```python
from build123d import *

# Parameters (mm, degrees)
SKETCH_1_R      = 8
SKETCH_1_R_2    = 1.56
EXTRUDE_1_DEPTH = 3


with BuildPart() as part:
    # 草图1 → 凸台-拉伸1 (new body)
    with BuildSketch(Plane.XY):
        with BuildLine():
            Line((-27.357864376, 42), (27.357864376, 42))
            ThreePointArc((27.357864376, 42), (31.1846987, 41.238795325), (34.428932188, 39.071067812))
            Line((34.428932188, 39.071067812), (39.071067812, 34.428932188))
            ThreePointArc((39.071067812, 34.428932188), (41.238795325, 31.1846987), (42, 27.357864376))
            Line((42, 27.357864376), (42, -27.357864376))
            ThreePointArc((42, -27.357864376), (41.238795325, -31.1846987), (39.071067812, -34.428932188))
            Line((39.071067812, -34.428932188), (34.428932188, -39.071067812))
            ThreePointArc((34.428932188, -39.071067812), (31.1846987, -41.238795325), (27.357864376, -42))
            Line((27.357864376, -42), (-27.357864376, -42))
            ThreePointArc((-27.357864376, -42), (-31.1846987, -41.238795325), (-34.428932188, -39.071067812))
            Line((-34.428932188, -39.071067812), (-39.071067812, -34.428932188))
            ThreePointArc((-39.071067812, -34.428932188), (-41.238795325, -31.1846987), (-42, -27.357864376))
            Line((-42, -27.357864376), (-42, 27.357864376))
            ThreePointArc((-42, 27.357864376), (-41.238795325, 31.1846987), (-39.071067812, 34.428932188))
            Line((-39.071067812, 34.428932188), (-34.428932188, 39.071067812))
            ThreePointArc((-34.428932188, 39.071067812), (-31.1846987, 41.238795325), (-27.357864376, 42))
        make_face()
        Circle(SKETCH_1_R, mode=Mode.SUBTRACT)
        with Locations((-26.196699141, 36.803300859)):
            Circle(SKETCH_1_R_2, mode=Mode.SUBTRACT)
        with Locations((-36.803300859, 26.196699141)):
            Circle(SKETCH_1_R_2, mode=Mode.SUBTRACT)
        with Locations(Location((26.196699141, 36.803300859, 0), (0, 0, 180))):
            Circle(SKETCH_1_R_2, mode=Mode.SUBTRACT)
        with Locations(Location((36.803300859, 26.196699141, 0), (0, 0, 180))):
            Circle(SKETCH_1_R_2, mode=Mode.SUBTRACT)
        with Locations((36.803300859, -26.196699141)):
            Circle(SKETCH_1_R_2, mode=Mode.SUBTRACT)
        with Locations((26.196699141, -36.803300859)):
            Circle(SKETCH_1_R_2, mode=Mode.SUBTRACT)
        with Locations(Location((-26.196699141, -36.803300859, 0), (0, 0, 180))):
            Circle(SKETCH_1_R_2, mode=Mode.SUBTRACT)
        with Locations(Location((-36.803300859, -26.196699141, 0), (0, 0, 180))):
            Circle(SKETCH_1_R_2, mode=Mode.SUBTRACT)
        with Locations((0, 36.803300859)):
            Circle(SKETCH_1_R_2, mode=Mode.SUBTRACT)
        with Locations(Location((36.803300859, 0, 0), (0, 0, 180))):
            Circle(SKETCH_1_R_2, mode=Mode.SUBTRACT)
        with Locations(Location((0, -36.803300859, 0), (0, 0, 180))):
            Circle(SKETCH_1_R_2, mode=Mode.SUBTRACT)
        with Locations((-36.803300859, 0)):
            Circle(SKETCH_1_R_2, mode=Mode.SUBTRACT)
        with BuildLine():
            Line((-17.5, 24.05), (17.5, 24.05))
            ThreePointArc((17.5, 24.05), (19.05, 22.5), (17.5, 20.95))
            Line((17.5, 20.95), (-17.5, 20.95))
            ThreePointArc((-17.5, 20.95), (-19.05, 22.5), (-17.5, 24.05))
        make_face(mode=Mode.SUBTRACT)
        with BuildLine():
            Line((-17.5, -24.05), (17.5, -24.05))
            ThreePointArc((17.5, -24.05), (19.05, -22.5), (17.5, -20.95))
            Line((17.5, -20.95), (-17.5, -20.95))
            ThreePointArc((-17.5, -20.95), (-19.05, -22.5), (-17.5, -24.05))
        make_face(mode=Mode.SUBTRACT)
        with BuildLine():
            Line((24.05, -17.5), (24.05, 17.5))
            ThreePointArc((24.05, 17.5), (22.5, 19.05), (20.95, 17.5))
            Line((20.95, 17.5), (20.95, -17.5))
            ThreePointArc((20.95, -17.5), (22.5, -19.05), (24.05, -17.5))
        make_face(mode=Mode.SUBTRACT)
        with BuildLine():
            Line((-24.05, -17.5), (-24.05, 17.5))
            ThreePointArc((-24.05, 17.5), (-22.5, 19.05), (-20.95, 17.5))
            Line((-20.95, 17.5), (-20.95, -17.5))
            ThreePointArc((-20.95, -17.5), (-22.5, -19.05), (-24.05, -17.5))
        make_face(mode=Mode.SUBTRACT)
        with BuildLine():
            Line((8.903984489, 11.096015511), (13.903984489, 16.096015511))
            ThreePointArc((13.903984489, 16.096015511), (16.096015511, 16.096015511), (16.096015511, 13.903984489))
            Line((16.096015511, 13.903984489), (11.096015511, 8.903984489))
            ThreePointArc((11.096015511, 8.903984489), (8.903984489, 8.903984489), (8.903984489, 11.096015511))
        make_face(mode=Mode.SUBTRACT)
        with BuildLine():
            Line((-8.903984489, 11.096015511), (-13.903984489, 16.096015511))
            ThreePointArc((-13.903984489, 16.096015511), (-16.096015511, 16.096015511), (-16.096015511, 13.903984489))
            Line((-16.096015511, 13.903984489), (-11.096015511, 8.903984489))
            ThreePointArc((-11.096015511, 8.903984489), (-8.903984489, 8.903984489), (-8.903984489, 11.096015511))
        make_face(mode=Mode.SUBTRACT)
        with BuildLine():
            Line((-8.903984489, -11.096015511), (-13.903984489, -16.096015511))
            ThreePointArc((-13.903984489, -16.096015511), (-16.096015511, -16.096015511), (-16.096015511, -13.903984489))
            Line((-16.096015511, -13.903984489), (-11.096015511, -8.903984489))
            ThreePointArc((-11.096015511, -8.903984489), (-8.903984489, -8.903984489), (-8.903984489, -11.096015511))
        make_face(mode=Mode.SUBTRACT)
        with BuildLine():
            Line((8.903984489, -11.096015511), (13.903984489, -16.096015511))
            ThreePointArc((13.903984489, -16.096015511), (16.096015511, -16.096015511), (16.096015511, -13.903984489))
            Line((16.096015511, -13.903984489), (11.096015511, -8.903984489))
            ThreePointArc((11.096015511, -8.903984489), (8.903984489, -8.903984489), (8.903984489, -11.096015511))
        make_face(mode=Mode.SUBTRACT)
    extrude(amount=EXTRUDE_1_DEPTH)


solid = part.part
```
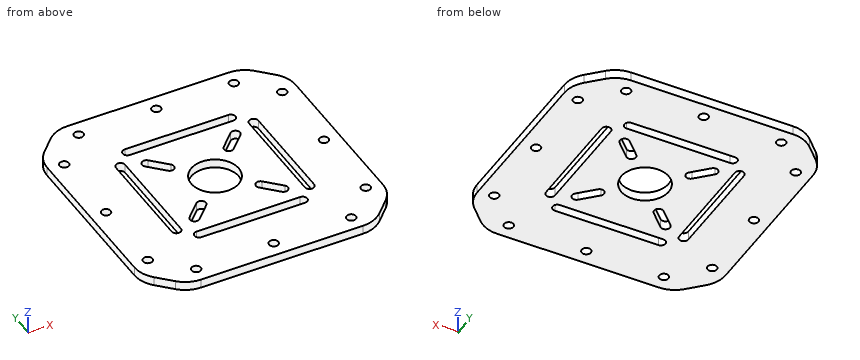
Could you check a few things on this model? Use its own coordinates, in mm. Round coordinates to 2 decimals unless told otherwise and drop trailing zeros. Loops run counter-clockwise (first coordinate to the right, second up) from the corner with the lowest first, then second, coordinate; pieces in that order, holes last. Notation, with made-up numbers: (-15.75, -22.75) - (-5.75, -22.75) arc R25 ccw to (-5.75, -10.75) - close; hole circle Ø6 at (38.25, -39). An arc over 180 degrees is marked (long way). Use CSV: the item, a comma, the result in double quotes.
Item 1: If we section it at D-D on x = -10: List the corners of the cut face in (y, z) for me, then the cut area to 3 significant figures.
Here are the results:
outline,"(-42, 0) - (-24.05, 0) - (-24.05, 3) - (-42, 3) - close; (-20.95, 0) - (-12.19, 0) - (-12.19, 3) - (-20.95, 3) - close; (-8.45, 0) - (8.45, 0) - (8.45, 3) - (-8.45, 3) - close; (12.19, 0) - (20.95, 0) - (20.95, 3) - (12.19, 3) - close; (24.05, 0) - (42, 0) - (42, 3) - (24.05, 3) - close"
area,"211 mm²"
Item 2: If we section it at A-A on x = 0: List the corners of the cut face in (y, z) for me.
Here are the results:
outline,"(-42, 0) - (-38.36, 0) - (-38.36, 3) - (-42, 3) - close; (-35.24, 0) - (-24.05, 0) - (-24.05, 3) - (-35.24, 3) - close; (-20.95, 0) - (-8, 0) - (-8, 3) - (-20.95, 3) - close; (8, 0) - (20.95, 0) - (20.95, 3) - (8, 3) - close; (24.05, 0) - (35.24, 0) - (35.24, 3) - (24.05, 3) - close; (38.36, 0) - (42, 0) - (42, 3) - (38.36, 3) - close"
Item 3: I need wall thicknesses on L1, parallel to Y at x = 0, z = 1.6; L2, parallel to Y at x = 27, z = 1.3; L3, parallel to Y at x = -26.5, z = 1.5. Which ranges of each line are inside material? Lowest first, please. Write a range as [from, to].
Here are the results:
L1,"y = [-42, -38.36], [-35.24, -24.05], [-20.95, -8], [8, 20.95], [24.05, 35.24], [38.36, 42]"
L2,"y = [-42, -38.14], [-35.47, 35.47], [38.14, 42]"
L3,"y = [-42, -38.33], [-35.27, 35.27], [38.33, 42]"
Item 4: If we section it at C-C on y = 12.5: List the corners of the cut face in (x, z) for me.
Here are the results:
outline,"(-42, 0) - (-24.05, 0) - (-24.05, 3) - (-42, 3) - close; (-20.95, 0) - (-14.69, 0) - (-14.69, 3) - (-20.95, 3) - close; (-10.31, 0) - (10.31, 0) - (10.31, 3) - (-10.31, 3) - close; (14.69, 0) - (20.95, 0) - (20.95, 3) - (14.69, 3) - close; (24.05, 0) - (42, 0) - (42, 3) - (24.05, 3) - close"
Item 5: Will this pin go through, and if not, where does the flat tip stop? pin 1 (3 mm diameter, centred on x = -36.8, y = -26.2, fed in from +Z).
Here are the results:
pin 1,"passes through"
